The listing builds one solid part. Answer for the finished solid, in the listing's coordinates (mm). A direction names the side the tool comes from. Give positions to 0.01 mm unless a question says otherwise; leave off trailing zeros. Write each loop counter-clockwise with the first axis right and the second up, starting at its lowest first coordinate (ties: lowest second). Pieces come first, ordered by that corner, then holes. Notation, with made-up numbers: (1.5, -38) -> (9.5, -38) arc R35 ccw to (9.5, -5) -> close; hole circle Ø5 at (41.5, 13.25). An arc over 180 degrees is marked (long way). One line per question, with ' | ' between items.
from build123d import *

# Parameters (mm, degrees)
SKETCH_1_R          = 5
SKETCH_1_R_2        = 1.6
EXTRUDE_1_DEPTH     = 15
CUT_EXTRUDE_1_DEPTH = 2.5
SKETCH_4_R          = 2.5
SKETCH_4_R_2        = 1.6
EXTRUDE_2_DEPTH     = 7


with BuildPart() as part:
    # 草图1 → 凸台-拉伸1 (new body)
    with BuildSketch(Plane.XY):
        Circle(SKETCH_1_R)
        Circle(SKETCH_1_R_2, mode=Mode.SUBTRACT)
    extrude(amount=EXTRUDE_1_DEPTH)

    # 草图2 → 切除-拉伸1 (cut)
    with BuildSketch(Plane.XY.offset(15)):
        Polygon((3.4, 0), (1.7, 2.944486373), (-1.7, 2.944486373), (-3.4, 0), (-1.7, -2.944486373), (1.7, -2.944486373), align=None)
    extrude(amount=-CUT_EXTRUDE_1_DEPTH, mode=Mode.SUBTRACT)

    # 草图4 → 凸台-拉伸2 (add)
    with BuildSketch(Plane(origin=(0, 4, 0), x_dir=(1, 0, 0), z_dir=(0, 1, 0))):
        with Locations(Location((0, -2.5, 0), (0, 0, 270))):
            Circle(SKETCH_4_R)
        with Locations(Location((0, -2.5, 0), (0, 0, 90))):
            Circle(SKETCH_4_R_2, mode=Mode.SUBTRACT)
    extrude(amount=EXTRUDE_2_DEPTH)


solid = part.part
Item 1: Find section C-C (y = 9.5). Write down the section's boundary in (x, z), then the cut area to 3 significant figures.
Answers below:
outline: circle Ø5 at (0, 2.5); hole circle Ø3.2 at (0, 2.5) | area: 11.6 mm²
Item 2: Determine the mould class of faces 1 (the face through (-1.08, -4.88, 7.39)), 2 (the face through (2, 0, 0)), 3 (the face through (0, -2.944, 14)) for opening direction Y: pulls with the +Y half, pulls with the -Y half, needs draft (parallel to the pull), parting line crosses it, or undercut.
Answers below:
face 1: parting line crosses it | face 2: needs draft | face 3: undercut
Item 3: Consider line 1 (X direction, y = 8.5, z = 2.5); line 2 (X direction, y = 0, z = 8). Determine where each line is inside the solid, lowest interval first. Write a range as [from, to].
Answers below:
line 1: [-2.5, -1.6], [1.6, 2.5] | line 2: [-5, -1.6], [1.6, 5]
Item 4: Find section B-B (x = -0.75). Write down the section's boundary in (y, z).
Answers below:
outline: (-4.94, 0) -> (-1.41, 0) -> (-1.41, 12.5) -> (-2.94, 12.5) -> (-2.94, 15) -> (-4.94, 15) -> close; (1.41, 0) -> (4.94, 0) -> (4.94, 0.12) -> (11, 0.12) -> (11, 1.09) -> (4.94, 1.09) -> (4.94, 3.91) -> (11, 3.91) -> (11, 4.88) -> (4.94, 4.88) -> (4.94, 15) -> (2.94, 15) -> (2.94, 12.5) -> (1.41, 12.5) -> close
Item 5: Find section D-D (x = 2). Write down the section's boundary in (y, z), then the cut area to 3 significant figures.
Answers below:
outline: (-4.58, 0) -> (4.58, 0) -> (4.58, 1) -> (11, 1) -> (11, 4) -> (4.58, 4) -> (4.58, 15) -> (2.42, 15) -> (2.42, 12.5) -> (-2.42, 12.5) -> (-2.42, 15) -> (-4.58, 15) -> close | area: 145 mm²
Item 6: A flat-ended cylindrical pin translates along its axis: pin 1 (2 mm diameter, centred on x = 0, z = 14, fed in from +Y). Find the tip coordinate at first contact, or state that the pin passes through.
Answers below:
pin 1: y = 5
Item 7: Find section A-A (z = 2.5). Write down the section's boundary in (x, y), then the cut area to 3 significant figures.
Answers below:
outline: (-2.5, 4.33) arc R5 ccw (long way) to (2.5, 4.33) -> (2.5, 11) -> (1.6, 11) -> (1.6, 4.74) arc R5 ccw to (-1.6, 4.74) -> (-1.6, 11) -> (-2.5, 11) -> close; hole circle Ø3.2 at (0, 0) | area: 82.1 mm²
Item 8: A tool of negligible diameter and unlimited length cuts with its end or side. For faces 4 (the face through (-2.562, -1.452, 13.768)), 5 (the face through (-1.27, -0.97, 6.16)), 6 (the face through (0.61, 7.82, 1.02)), from which of +Z, -Z, +X, -X, +Y, -Y can it reach the whole face along a straight path? Write none if from no direction.
Answers below:
face 4: +Z | face 5: +Z, -Z | face 6: +Y
